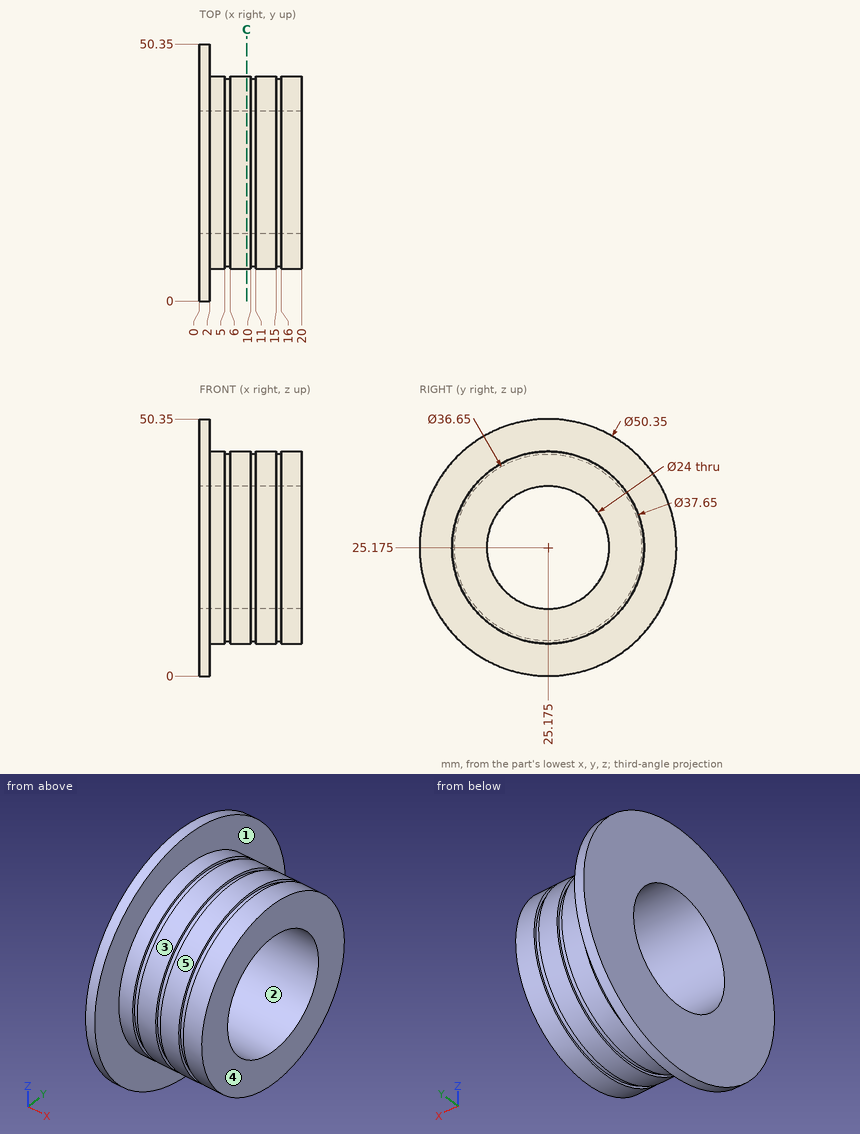
Design review of the part shown in the three views and the two pictorial views. Dimensions are in mm from the part's minimum x, y and z. A direction names the side the tool comes from. Give positions to 0.01 mm unless a question says otherwise; leave off trailing zeros. Order: outer loops, then holes, each group sorted by start corner. A loop starts at its lowest first (then second) coordinate and runs counter-clockwise, first axis right, second up. Notation, with made-up numbers: M 21,-28.75 L 56,-28.75 A32 ccw 56,-1.75 Z; hole C -14.75,86 d4. An arc over 180 degrees is marked long. Answer in a Markdown table with one row per item. Add a question column.
(1) Mouldability with a two-part tool opening along Z and no side actions: class the marked faces 1, 2 and 3 as +Z half, -Z half, draft (parallel to the pull), parting line (faces both ways), or undercut.
(2) For the marked faces 4 and 5, list the 3-axis set-ups (+Z, -Z, +X, -X, +Y, -Y) from which the entire face can be reached by the end or side of a thin tool; tool diameter is ignored.
(3) Wall thickness on probe 1 along X at (y, z) = (45.5, 33.5); probe 2 along Y at (x, z) = (3.75, 34); probe 3 along Y at (x, z) = (15.75, 18): over which ranges is each line inside the solid? List them lowest first. Write a range as [from, to].
(4) For pin 1 (8 mm diameter, centred on x = 10.5, z = 28, fed in from -Y); pin 2 (10 mm diameter, centred on x = 3, y = 23.5, fed in from +Z); pin 3 (2 mm diameter, centred on x = 8.5, y = 38, fed in from +Z); pin 4 (12 mm diameter, centred on x = 14.5, y = 41, fed in from +Z), all flat-tipped, find the tip position at first contact; note any pin that passes through.
(5) Consider section C-C on x = 9.25. State the section outline as (y, z) points (3 decimals), and give its area (3 significant figures).
Evaluation:
| question | item | result |
|---|---|---|
| 1 | face 1 | draft |
| 1 | face 2 | undercut |
| 1 | face 3 | parting line |
| 2 | face 4 | +Z, -Z, +X, +Y, -Y |
| 2 | face 5 | +X |
| 3 | probe 1 | x = [0, 2] |
| 3 | probe 2 | y = [8.55, 17.04], [33.31, 41.8] |
| 3 | probe 3 | y = [8.31, 15.56], [34.79, 42.04] |
| 4 | pin 1 | stops at y = 6.35 |
| 4 | pin 2 | stops at z = 50.35 |
| 4 | pin 3 | stops at z = 39.82 |
| 4 | pin 4 | stops at z = 41.23 |
| 5 | outline | C 25.175,25.175 d37.65; hole C 25.175,25.175 d24 |
| 5 | area | 661 mm^2 |
